The listing builds one solid part. Answer for the finished solid, in the listing's coordinates (mm). A direction names the side the tool comes from. Coordinates: 2 decimals unless noted, no trailing zeros. Order: outer loops, then holes, each group sorted by start corner. A loop starts at its lowest first (then second) coordinate and runs counter-clockwise, first axis right, second up. Notation, with made-up numbers: (13.5, 45) -> (55.5, 45) arc R18 ccw to (55.5, 73) -> close; hole circle Ø5 at (4.25, 66). An arc over 180 degrees is marked (long way). Write each question's results on one line, items separated by ' | '. Start each with the question number.
(1) The part is cut by section D-D, the plane z = 0. Give the vertices of the cut face in (x, y).
(2) Given pin 1 (20 mm diameter, centred on x = 38, z = 9.5, fed in from +Y); pin 2 (3 mm diameter, centred on y = 9, z = -13, fed in from -X); pin 3 (11 mm diameter, centred on y = 20.5, z = -14, fed in from +X), each flat-ended and moving along its own axis, determine where each tip first touches the part or whether it passes through.
(3) Determine the mould class of faces 5 (the face through (3.01, 0.07, 17.15)), 6 (the face through (84.619, 1.056, 1.915)), 7 (the face through (49, -5, -15)), 8 (the face through (15, 1, 0)) for opening direction Z: +Z half, -Z half, draft (parallel to the pull), parting line (faces both ways), or undercut.
(4) The part is cut by section B-B, the plane x = 50. Give the vertices of the cut face in (y, z), then the cut area to 3 significant figures.
(5) The part is cut by section C-C, the plane x = 87. Give the vertices of the cut face in (y, z), then the cut area to 3 significant figures.
(6) Straight lines are drawn through the part: L1, parallel to X at y = 0.5, z = 0; L2, parallel to Z at x = 20, y = -0.25; L3, parallel to Z at x = 57, y = 49. For each, find the intervals that lie inside material, in ascending order.
(7) A tool of negligible diameter and unlimited length cuts with its end or side. For faces 1 (the face through (51, -4, 10)), 2 (the face through (70, 24, -15)), 3 (the face through (30, 24, -15)), 4 (the face through (50, 24, -10)), from which of +Z, -Z, +X, -X, +Y, -Y can it reach the whole face along a straight path? Write none if from no direction.
(8) The part is cut by section A-A, the plane z = -15. Give the vertices of the cut face in (x, y), then the cut area to 3 significant figures.
```python
from build123d import *

# Parameters (mm, degrees)
CROQUIS1_W              = 40
CROQUIS1_H              = 10
SALIENTE_EXTRUIR1_DEPTH = 100
REDONDEO2_R             = 10
CROQUIS2_W              = 20
CROQUIS2_H              = 2
CORTAR_EXTRUIR1_DEPTH   = 100
CROQUIS3_R              = 5
CORTAR_EXTRUIR2_DEPTH   = 10
CROQUIS5_R              = 7.5
SALIENTE_EXTRUIR3_DEPTH = 10


with BuildPart() as part:
    # Croquis1 → Saliente-Extruir1 (new body)
    with BuildSketch(Plane(origin=(0, 0, 0), x_dir=(0, 0, -1), z_dir=(1, 0, 0))):
        Rectangle(CROQUIS1_W, CROQUIS1_H)
    extrude(amount=SALIENTE_EXTRUIR1_DEPTH)

    # Redondeo2
    redondeo2_edges = [part.edges().sort_by_distance(p)[0] for p in [
        (100, 0, 20),
        (0, 0, 20),
    ]]
    fillet(redondeo2_edges, radius=REDONDEO2_R)

    # Croquis2 → Cortar-Extruir1 (cut)
    with BuildSketch(Plane(origin=(100, 0, 0), x_dir=(0, 0, -1), z_dir=(1, 0, 0))):
        with Locations((0, -4)):
            Rectangle(CROQUIS2_W, CROQUIS2_H)
    extrude(amount=-CORTAR_EXTRUIR1_DEPTH, mode=Mode.SUBTRACT)

    # Croquis3 → Cortar-Extruir2 (cut)
    with BuildSketch(Plane(origin=(0, 5, 0), x_dir=(1, 0, 0), z_dir=(0, 1, 0))):
        with Locations((20, 0)):
            Circle(CROQUIS3_R)
        with Locations((80, 0)):
            Circle(CROQUIS3_R)
    extrude(amount=-CORTAR_EXTRUIR2_DEPTH, mode=Mode.SUBTRACT)

    # Croquis5 → Saliente-Extruir3 (add)
    with BuildSketch(Plane(origin=(0, 0, -20), x_dir=(-1, 0, 0), z_dir=(0, 0, -1))):
        with BuildLine():
            Line((-70, 32.5), (-70, 15))
            ThreePointArc((-70, 15), (-72.928932188, 7.928932188), (-80, 5))
            Line((-80, 5), (-20, 5))
            ThreePointArc((-20, 5), (-27.071067812, 7.928932188), (-30, 15))
            Line((-30, 15), (-30, 32.5))
            ThreePointArc((-30, 32.5), (-50, 52.5), (-70, 32.5))
        make_face()
        with Locations((-50, 32.5)):
            Circle(CROQUIS5_R, mode=Mode.SUBTRACT)
    extrude(amount=-SALIENTE_EXTRUIR3_DEPTH)


solid = part.part
```
Established:
1) outline: (0, -3) -> (15, -3) -> (15, 5) -> (0, 5) -> close; (25, -3) -> (75, -3) -> (75, 5) -> (25, 5) -> close; (85, -3) -> (100, -3) -> (100, 5) -> (85, 5) -> close
2) pin 1: stops at y = 5 | pin 2: stops at x = 26.61 | pin 3: stops at x = 70
3) face 5: +Z half | face 6: undercut | face 7: draft | face 8: undercut
4) outline: (-5, -20) -> (25, -20) -> (25, -10) -> (5, -10) -> (5, 20) -> (-5, 20) -> (-5, 10) -> (-3, 10) -> (-3, -10) -> (-5, -10) -> close; (40, -20) -> (52.5, -20) -> (52.5, -10) -> (40, -10) -> close | area: 685 mm^2
5) outline: (-5, -20) -> (5, -20) -> (5, 20) -> (-5, 20) -> (-5, 10) -> (-3, 10) -> (-3, -10) -> (-5, -10) -> close | area: 360 mm^2
6) L1: x = 0 to 15, 25 to 75, 85 to 100 | L2: z = -20 to -5, 5 to 20 | L3: z = -20 to -10
7) face 1: +X, -X, -Y | face 2: +Z, -Z, +X, +Y | face 3: +Z, -Z, -X, +Y | face 4: +Z, +X, -X, +Y
8) outline: (0, -5) -> (100, -5) -> (100, 5) -> (80, 5) arc R10 cw to (70, 15) -> (70, 32.5) arc R20 ccw to (30, 32.5) -> (30, 15) arc R10 cw to (20, 5) -> (0, 5) -> close; hole circle Ø15 at (50, 32.5) | area: 2,590 mm^2
